Geometry: final body of the model. Coordinates: model frame, mm. A direction names the side the tool comes from. Coordinates: 2 decimals unless noted, no trailing zeros. Order: outer loops, then holes, each group sorted by start corner. A loop starts at its lowest first (then second) coordinate and runs counter-clockwise, first axis right, second up. Notation, with made-up numbers: M -6,2 L 31,2 A15 ccw 31,31 Z; hole C -8.75,11 d8. An arc over 180 degrees is marked long. One line per question, with ' | ' between items.
from build123d import *

# Parameters (mm, degrees)
SKETCH3_R          = 0.508
CUT_EXTRUDE1_DEPTH = 3.54


with BuildPart() as part:
    # Sketch2 → Revolve1 (revolve)
    with BuildSketch(Plane.XY):
        with BuildLine():
            Line((0.889, 12.7), (-0.889, 12.7))
            ThreePointArc((-0.889, 12.7), (-1.60742049, 12.40242049), (-1.905, 11.684))
            Line((-1.905, 11.684), (-1.905, 11.176))
            ThreePointArc((-1.905, 11.176), (-1.60742049, 10.45757951), (-0.889, 10.16))
            Line((-0.889, 10.16), (-0.635, 10.16))
            Line((-0.635, 10.16), (-0.635, 0))
            Line((-0.635, 0), (0.635, 0))
            Line((0.635, 0), (0.635, 10.16))
            Line((0.635, 10.16), (0.889, 10.16))
            ThreePointArc((0.889, 10.16), (1.60742049, 10.45757951), (1.905, 11.176))
            Line((1.905, 11.176), (1.905, 11.684))
            ThreePointArc((1.905, 11.684), (1.60742049, 12.40242049), (0.889, 12.7))
        make_face()
    revolve(axis=Axis((-0.635, 0, 0), (1, 0, 0)))

    # Sketch3 → Cut-Extrude1 (cut, through all)
    with BuildSketch(Plane(origin=(0.635, 0, 0), x_dir=(0, 0, -1), z_dir=(1, 0, 0))):
        Circle(SKETCH3_R)
    extrude(amount=-CUT_EXTRUDE1_DEPTH, mode=Mode.SUBTRACT)


solid = part.part
1. Pin query (flat end, axial travel): P1, Ø3, axis at y = -2.5, z = -3, coming from the +X side (3 decimals); P2, Ø6, axis at y = -1, z = 0.5, coming from the -X side (3 decimals); P3, Ø1.5, axis at x = 0, z = -4, coming from the +Y side. Return the tip coordinate at first contact, or that it passes through.
Response values:
P1: stops at x = 0.635 | P2: stops at x = -0.635 | P3: stops at y = 12.28
2. Material intervals for line 1 (Z direction, x = -0.7, y = 0); line 2 (X direction, y = 0.5, z = -1) (3 decimals); line 3 (Y direction, x = -1.45, z = 2.5), sorted ascending. Write a range as [from, to].
Response values:
line 1: z = [-12.7, -10.16], [10.16, 12.7] | line 2: x = [-0.635, 0.635] | line 3: y = [-12.28, -10.02], [10.02, 12.28]
3. Section C-C, the plane x = 0.3. Output: boundary loops of the cut face in (y, z).
Response values:
outline: C 0,0 d25.4; hole C 0,0 d1.02
4. Access query for faces 3 (the face through (0.635, 0, -2)), 4 (the face through (-0.635, 0, -2)). Directions: +Z, -Z, +X, -X, +Y, -Y. A direction counts if a zero-diameter tool reaches every point of the face in a straight line with its end or side. Return the directions, or none.
Response values:
face 3: +X | face 4: -X
5. Draft query along Z for faces 1 (the face through (0, -0.5, 0.1)), 2 (the face through (-0.01, -2.75, -12.4)). Return one class per face: pulls with the +Z half, pulls with the -Z half, needs draft (parallel to the pull), parting line crosses it, or undercut.
Response values:
face 1: undercut | face 2: parting line crosses it
6. Section A-A, the plane y = 0. Output: boundary loops of the cut face in (x, z) (3 decimals), and give its area (3 significant figures).
Response values:
outline: M -1.905,-11.684 A1.016 ccw -0.889,-12.7 L 0.889,-12.7 A1.016 ccw 1.905,-11.684 L 1.905,-11.176 A1.016 ccw 0.889,-10.16 L 0.635,-10.16 L 0.635,-0.508 L -0.635,-0.508 L -0.635,-10.16 L -0.889,-10.16 A1.016 ccw -1.905,-11.176 Z; M -1.905,11.176 A1.016 ccw -0.889,10.16 L -0.635,10.16 L -0.635,0.508 L 0.635,0.508 L 0.635,10.16 L 0.889,10.16 A1.016 ccw 1.905,11.176 L 1.905,11.684 A1.016 ccw 0.889,12.7 L -0.889,12.7 A1.016 ccw -1.905,11.684 Z | area: 42.1 mm^2
